Build history of the part. All positions in model axes, mm. A direction names the side the tool comes from. Round coordinates to 2 decimals unless told otherwise and drop trailing zeros. Loops run counter-clockwise (first coordinate to the right, second up) from the corner with the lowest first, then second, coordinate; pieces in that order, holes last. Notation, with made-up numbers: M -2.75,26.25 L 24.25,26.25 A17 cw 24.25,56.25 Z; hole C -40,-7.5 d7. An arc over 180 degrees is marked long. Write each question's results on one line, items separated by ' | '. Start each with the question number.
```python
from build123d import *

# Parameters (mm, degrees)
SKETCH1_R           = 57.5
SKETCH1_R_2         = 52.5
BOSS_EXTRUDE1_DEPTH = 32
SKETCH3_R           = 52.5
SKETCH3_R_2         = 45
SKETCH3_R_3         = 35
BOSS_EXTRUDE3_DEPTH = 12
SKETCH7_R           = 45
SKETCH7_R_2         = 42.5
BOSS_EXTRUDE4_DEPTH = 2
SKETCH10_R          = 52.5
SKETCH10_R_2        = 43
BOSS_EXTRUDE5_DEPTH = 3


with BuildPart() as part:
    # Sketch1 → Boss-Extrude1 (new body)
    with BuildSketch(Plane.XY):
        Circle(SKETCH1_R)
        Circle(SKETCH1_R_2, mode=Mode.SUBTRACT)
    extrude(amount=BOSS_EXTRUDE1_DEPTH)

    # Sketch3 → Boss-Extrude3 (add)
    # profile 1 of 2: a face of its own
    with BuildSketch(Plane.XY.offset(20)):
        Circle(SKETCH3_R)
        Circle(SKETCH3_R_2, mode=Mode.SUBTRACT)
    # profile 2 of 2: a face of its own
    with BuildSketch(Plane.XY.offset(20)):
        Circle(SKETCH3_R_3)
    extrude(amount=BOSS_EXTRUDE3_DEPTH)


with BuildPart() as boss_extrude3_kept_piece:
    # of the separate pieces the step leaves, the one the design keeps (boss_extrude3_pieces_kept)
    add(part.part.solids().sort_by_distance((57.5, 0, 0))[0])

    # Sketch7 → Boss-Extrude4 (add)
    with BuildSketch(Plane.XY.offset(20)):
        Circle(SKETCH7_R)
        Circle(SKETCH7_R_2, mode=Mode.SUBTRACT)
    extrude(amount=BOSS_EXTRUDE4_DEPTH)

    # Sketch10 → Boss-Extrude5 (add)
    with BuildSketch(Plane(origin=(0, 0, 0), x_dir=(-1, 0, 0), z_dir=(0, 0, -1))):
        Circle(SKETCH10_R)
        Circle(SKETCH10_R_2, mode=Mode.SUBTRACT)
    extrude(amount=-BOSS_EXTRUDE5_DEPTH)


solid = boss_extrude3_kept_piece.part
```
Item 1: Saw through at D-D, the plane y = -48.5. Give the cut face in (x, z), then the cut area to 3 significant figures.
Item 2: Tool access for faces 4 (the cylindrical face through (5.598, 42.634, 1.479)), 5 (the cylindrical face through (20.765, -39.923, 26.93)), 6 (the flat face through (43, 0, 20)): list every direction of +Z, -Z, +X, -X, +Y, -Y with a clear straight run to the whole face (end or side of a thin tool).
Item 3: Saw through at C-C, the plane z = 13. Give the cut face in (x, y), then the cut area to 3 significant figures.
Item 4: Saw through at A-A, the plane y = 0. Give the cut face in (x, z).
Item 5: Mould opens along X. For faces 1 (the cylindrical face through (-12.465, -56.133, 15.776)), 2 (the flat face through (-34, -30, 32)), 3 (the flat face through (20, -39, 3)) say: released by +X, released by -X, zero draft, split by the parting line, or undercut.
Item 6: Drop flat-ended pins along their axis: pin 1 (1 mm diameter, centred on y = 7.5, z = 13, fed in from -X); pin 2 (8 mm diameter, centred on y = 5.5, z = 15.5, fed in from -X); pin 3 (6 mm diameter, centred on x = 4.5, z = 25.5, fed in from -Y). Give the stop position or say it passes through.
Item 7: Drill centre lines: line 1 along Y through (x, z) = (0, 21.45); line 2 along Z through (x, y) = (-24, -38); line 3 along Y through (x, z) = (0, 0.85). Where is each one in solid material? Low to high. Write a range as [from, to].
Working result:
1) outline: M -30.89,0 L 30.89,0 L 30.89,32 L -30.89,32 Z; hole M -20.1,3 L 20.1,3 L 20.1,20 L -20.1,20 Z | area: 1,290 mm²
2) face 4: -Z | face 5: +Z | face 6: none
3) outline: C 0,0 d115; hole C 0,0 d105 | area: 1,730 mm²
4) outline: M -57.5,0 L -43,0 L -43,3 L -52.5,3 L -52.5,20 L -42.5,20 L -42.5,22 L -45,22 L -45,32 L -57.5,32 Z; M 42.5,20 L 52.5,20 L 52.5,3 L 43,3 L 43,0 L 57.5,0 L 57.5,32 L 45,32 L 45,22 L 42.5,22 Z
5) face 1: split by the parting line | face 2: zero draft | face 3: undercut
6) pin 1: stops at x = -57.07 | pin 2: stops at x = -57.48 | pin 3: stops at y = -57.48
7) line 1: y = [-57.5, -42.5], [42.5, 57.5] | line 2: z = [0, 3], [20, 22] | line 3: y = [-57.5, -43], [43, 57.5]
